Could you check a few things on this model? Use its own coordinates, in mm. A direction names the side the tool comes from. Give positions to 0.01 mm unless a question says otherwise; leave off trailing zeros. Return JSON: item names as keys, results as strings. Group by question number.
```python
from build123d import *

# Parameters (mm, degrees)
SKETCH1_W                    = 106
SKETCH1_H                    = 106
MAINOUTLINE_DEPTH            = 1.6
SKETCH4_W                    = 11.7
SKETCH4_H                    = 11.7
RAILCUTOUTS_DEPTH            = 75.970394157
SKETCH13_W                   = 5.7
SKETCH13_H                   = 1.9
SKETCH13_W_2                 = 1.8
SKETCH13_H_2                 = 3
FILLETCUTOUTS_DEPTH          = 75.970394157
SMOOTHCORNER_DEPTH           = 10
MIRROR2_COPY_1_SKETCH_W      = 11.7
MIRROR2_COPY_1_SKETCH_H      = 11.7
MIRROR2_COPY_1_DEPTH         = 75.970394157
MIRROR2_COPY_2_SKETCH_W      = 5.7
MIRROR2_COPY_2_SKETCH_H      = 1.9
MIRROR2_COPY_2_SKETCH_W_2    = 1.8
MIRROR2_COPY_2_SKETCH_H_2    = 3
MIRROR2_COPY_2_DEPTH         = 75.970394157
MIRROR2_COPY_3_DEPTH         = 10
MIRROR2_COPY_4_SKETCH_W      = 11.7
MIRROR2_COPY_4_SKETCH_H      = 11.7
MIRROR2_COPY_4_DEPTH         = 75.970394157
MIRROR2_COPY_5_SKETCH_W      = 5.7
MIRROR2_COPY_5_SKETCH_H      = 1.9
MIRROR2_COPY_5_SKETCH_W_2    = 1.8
MIRROR2_COPY_5_SKETCH_H_2    = 3
MIRROR2_COPY_5_DEPTH         = 75.970394157
FILLET10_R                   = 0.5
M2_CLEARANCE_HOLE1_D         = 2.1
SKETCH16_W                   = 90
SKETCH16_H                   = 5.2
SKETCH16_W_2                 = 5.2
SKETCH16_H_2                 = 90
CUT_EXTRUDE6_DEPTH           = 0.001
CUT_EXTRUDE8_DEPTH           = 10
SKETCH29_R                   = 0.8
CONNECTOR_LOCATION_DEPTH     = 10
CUT_EXTRUDE_THIN1_DEPTH      = 75.970394157
CUT_EXTRUDE_THIN1_DEPTH_BACK = 75.970394157
SKETCH31_W                   = 125.6
SKETCH31_H                   = 125.6
SKETCH31_W_2                 = 105.6
SKETCH31_H_2                 = 105.6
FILLET12_R                   = 0.5


with BuildPart() as part:
    # Sketch1 → mainOutline (new body)
    with BuildSketch(Plane.XY):
        Rectangle(SKETCH1_W, SKETCH1_H)
    extrude(amount=MAINOUTLINE_DEPTH)

    # Sketch4 → railCutouts (cut, through all)
    with BuildSketch(Plane(origin=(0, 0, 0), x_dir=(-1, 0, 0), z_dir=(0, 0, -1))):
        with Locations((47.15, 47.15)):
            Rectangle(SKETCH4_W, SKETCH4_H)
    railcutouts = extrude(amount=-RAILCUTOUTS_DEPTH, mode=Mode.SUBTRACT)

    # Sketch13 → filletCutouts (cut, symmetric)
    with BuildSketch(Plane(origin=(0, 0, 0), x_dir=(-1, 0, 0), z_dir=(0, 0, -1))):
        with Locations((50.15, 40.35)):
            Rectangle(SKETCH13_W, SKETCH13_H)
        with Locations((40.4, 51.5)):
            Rectangle(SKETCH13_W_2, SKETCH13_H_2)
    filletcutouts = extrude(amount=FILLETCUTOUTS_DEPTH, both=True, mode=Mode.SUBTRACT)

    # Sketch27 → smoothCorner (cut)
    with BuildSketch(Plane.XY.offset(1.6)):
        with BuildLine():
            Line((-40.928025612, 42.198025612), (-40.928025612, 49.628025612))
            Line((-40.928025612, 49.628025612), (-40.398025612, 49.628025612))
            ThreePointArc((-40.398025612, 49.628025612), (-39.5, 50), (-39.128025612, 50.898025612))
            Line((-39.128025612, 50.898025612), (-39.128025612, 53))
            Line((-39.128025612, 53), (-53, 53))
            Line((-53, 53), (-53, 39.028025612))
            Line((-53, 39.028025612), (-48.198025612, 39.028025612))
            ThreePointArc((-48.198025612, 39.028025612), (-47.3, 39.4), (-46.928025612, 40.298025612))
            Line((-46.928025612, 40.298025612), (-46.928025612, 40.928025612))
            Line((-46.928025612, 40.928025612), (-42.198025612, 40.928025612))
            ThreePointArc((-42.198025612, 40.928025612), (-41.3, 41.3), (-40.928025612, 42.198025612))
        make_face()
    smoothcorner = extrude(amount=-SMOOTHCORNER_DEPTH, mode=Mode.SUBTRACT)

    # Mirror1: railCutouts, filletCutouts, smoothCorner across plane
    add(railcutouts.mirror(Plane(origin=(0, 0, 0), x_dir=(0, 0, 1), z_dir=(1, 0, 0))), mode=Mode.SUBTRACT)
    add(filletcutouts.mirror(Plane(origin=(0, 0, 0), x_dir=(0, 0, 1), z_dir=(1, 0, 0))), mode=Mode.SUBTRACT)
    add(smoothcorner.mirror(Plane(origin=(0, 0, 0), x_dir=(0, 0, 1), z_dir=(1, 0, 0))), mode=Mode.SUBTRACT)

    # Mirror2: smoothCorner across plane
    add(smoothcorner.mirror(Plane.ZX), mode=Mode.SUBTRACT)

    # Mirror2 copy 1 sketch → Mirror2 copy 1 (cut, through all)
    with BuildSketch(Plane(origin=(0, 0, 0), x_dir=(1, 0, 0), z_dir=(0, 0, -1))):
        with Locations((47.15, 47.15)):
            Rectangle(MIRROR2_COPY_1_SKETCH_W, MIRROR2_COPY_1_SKETCH_H)
    extrude(amount=-MIRROR2_COPY_1_DEPTH, mode=Mode.SUBTRACT)

    # Mirror2 copy 2 sketch → Mirror2 copy 2 (cut, symmetric)
    with BuildSketch(Plane(origin=(0, 0, 0), x_dir=(1, 0, 0), z_dir=(0, 0, -1))):
        with Locations((50.15, 40.35)):
            Rectangle(MIRROR2_COPY_2_SKETCH_W, MIRROR2_COPY_2_SKETCH_H)
        with Locations((40.4, 51.5)):
            Rectangle(MIRROR2_COPY_2_SKETCH_W_2, MIRROR2_COPY_2_SKETCH_H_2)
    extrude(amount=MIRROR2_COPY_2_DEPTH, both=True, mode=Mode.SUBTRACT)

    # Mirror2 copy 3 sketch → Mirror2 copy 3 (cut)
    with BuildSketch(Plane(origin=(0, 0, 1.6), x_dir=(-1, 0, 0), z_dir=(0, 0, 1))):
        with BuildLine():
            Line((-40.928025612, 42.198025612), (-40.928025612, 49.628025612))
            Line((-40.928025612, 49.628025612), (-40.398025612, 49.628025612))
            ThreePointArc((-40.398025612, 49.628025612), (-39.5, 50), (-39.128025612, 50.898025612))
            Line((-39.128025612, 50.898025612), (-39.128025612, 53))
            Line((-39.128025612, 53), (-53, 53))
            Line((-53, 53), (-53, 39.028025612))
            Line((-53, 39.028025612), (-48.198025612, 39.028025612))
            ThreePointArc((-48.198025612, 39.028025612), (-47.3, 39.4), (-46.928025612, 40.298025612))
            Line((-46.928025612, 40.298025612), (-46.928025612, 40.928025612))
            Line((-46.928025612, 40.928025612), (-42.198025612, 40.928025612))
            ThreePointArc((-42.198025612, 40.928025612), (-41.3, 41.3), (-40.928025612, 42.198025612))
        make_face()
    extrude(amount=-MIRROR2_COPY_3_DEPTH, mode=Mode.SUBTRACT)

    # Mirror2 copy 4 sketch → Mirror2 copy 4 (cut, through all)
    with BuildSketch(Plane(origin=(0, 0, 0), x_dir=(-1, 0, 0), z_dir=(0, 0, -1))):
        with Locations((47.15, -47.15)):
            Rectangle(MIRROR2_COPY_4_SKETCH_W, MIRROR2_COPY_4_SKETCH_H)
    extrude(amount=-MIRROR2_COPY_4_DEPTH, mode=Mode.SUBTRACT)

    # Mirror2 copy 5 sketch → Mirror2 copy 5 (cut, symmetric)
    with BuildSketch(Plane(origin=(0, 0, 0), x_dir=(-1, 0, 0), z_dir=(0, 0, -1))):
        with Locations((50.15, -40.35)):
            Rectangle(MIRROR2_COPY_5_SKETCH_W, MIRROR2_COPY_5_SKETCH_H)
        with Locations((40.4, -51.5)):
            Rectangle(MIRROR2_COPY_5_SKETCH_W_2, MIRROR2_COPY_5_SKETCH_H_2)
    extrude(amount=MIRROR2_COPY_5_DEPTH, both=True, mode=Mode.SUBTRACT)

    # Fillet10
    fillet10_edges = [part.edges().sort_by_distance(p)[0] for p in [
        (40.928025612, 49.628025612, 0.8),
        (46.928025612, 40.928025612, 0.8),
        (46.928025612, -40.928025612, 0.8),
        (40.928025612, -49.628025612, 0.8),
        (-40.928025612, -49.628025612, 0.8),
        (-46.928025612, -40.928025612, 0.8),
        (-46.928025612, 40.928025612, 0.8),
        (-40.928025612, 49.628025612, 0.8),
    ]]
    fillet(fillet10_edges, radius=FILLET10_R)

    # M2 Clearance Hole1 (through all)
    with Locations(Plane(origin=(0, 0, 0), x_dir=(-1, 0, 0), z_dir=(0, 0, -1))):
        with Locations((49.5, -27.5), (27.5, -49.5), (-49.5, -27.5), (-27.5, -49.5), (-27.5, 49.5), (-49.5, 27.5), (27.5, 49.5), (49.5, 27.5)):
            Hole(M2_CLEARANCE_HOLE1_D / 2)

    # Sketch16 → Cut-Extrude6 (cut)
    with BuildSketch(Plane.XY.offset(1.6)):
        with Locations((0, -50.4)):
            Rectangle(SKETCH16_W, SKETCH16_H)
        with Locations((0, 50.4)):
            Rectangle(SKETCH16_W, SKETCH16_H)
        with Locations((-50.4, 0)):
            Rectangle(SKETCH16_W_2, SKETCH16_H_2)
        with Locations((50.4, 0)):
            Rectangle(SKETCH16_W_2, SKETCH16_H_2)
    extrude(amount=-CUT_EXTRUDE6_DEPTH, mode=Mode.SUBTRACT)

    # Sketch30 → Cut-Extrude8 (cut)
    with BuildSketch(Plane(origin=(0, 0, 0), x_dir=(-1, 0, 0), z_dir=(0, 0, -1))):
        with BuildLine():
            Line((-18.930017367, -39.330048004), (-2.75, -23.150030637))
            Line((-2.75, -23.150030637), (2.75, -23.150030637))
            Line((2.75, -23.150030637), (18.930017367, -39.330048004))
            ThreePointArc((18.930017367, -39.330048004), (32.985735805, -32.985735805), (39.330048004, -18.930017367))
            Line((39.330048004, -18.930017367), (23.150030637, -2.75))
            Line((23.150030637, -2.75), (23.150030637, 2.75))
            Line((23.150030637, 2.75), (39.330048004, 18.930017367))
            ThreePointArc((39.330048004, 18.930017367), (32.985735805, 32.985735805), (18.930017367, 39.330048004))
            Line((18.930017367, 39.330048004), (2.75, 23.150030637))
            Line((2.75, 23.150030637), (-2.75, 23.150030637))
            Line((-2.75, 23.150030637), (-18.930017367, 39.330048004))
            ThreePointArc((-18.930017367, 39.330048004), (-32.985735805, 32.985735805), (-39.330048004, 18.930017367))
            Line((-39.330048004, 18.930017367), (-23.150030637, 2.75))
            Line((-23.150030637, 2.75), (-23.150030637, -2.75))
            Line((-23.150030637, -2.75), (-39.330048004, -18.930017367))
            ThreePointArc((-39.330048004, -18.930017367), (-32.985735805, -32.985735805), (-18.930017367, -39.330048004))
        make_face()
    extrude(amount=-CUT_EXTRUDE8_DEPTH, mode=Mode.SUBTRACT)

    # Sketch29 → Connector Location (cut)
    with BuildSketch(Plane(origin=(0, 0, 0), x_dir=(-1, 0, 0), z_dir=(0, 0, -1))):
        with Locations((34.285, -42.5)):
            Circle(SKETCH29_R)
        with Locations((23.515, -42.5)):
            Circle(SKETCH29_R)
    extrude(amount=-CONNECTOR_LOCATION_DEPTH, mode=Mode.SUBTRACT)

    # Sketch31 → Cut-Extrude-Thin1 (cut, two sides: drawn at the far end of the back side and taken through both)
    with BuildSketch(Plane(origin=(0, 0, 0), x_dir=(-1, 0, 0), z_dir=(0, 0, -1)).offset(-CUT_EXTRUDE_THIN1_DEPTH_BACK)):
        Rectangle(SKETCH31_W, SKETCH31_H)
        Rectangle(SKETCH31_W_2, SKETCH31_H_2, mode=Mode.SUBTRACT)
    extrude(amount=CUT_EXTRUDE_THIN1_DEPTH + CUT_EXTRUDE_THIN1_DEPTH_BACK, mode=Mode.SUBTRACT)

    # Fillet12
    fillet12_edges = [part.edges().sort_by_distance(p)[0] for p in [
        (-52.8, 39.028025612, 0.7995),
        (39.128025612, -52.8, 0.7995),
        (52.8, -39.028025612, 0.7995),
        (-39.128025612, 52.8, 0.7995),
        (-52.8, -39.028025612, 0.7995),
        (-39.128025612, -52.8, 0.7995),
        (52.8, 39.028025612, 0.7995),
        (39.128025612, 52.8, 0.7995),
    ]]
    fillet(fillet12_edges, radius=FILLET12_R)


solid = part.part
```
1. I need wall thicknesses on L1, parallel to Y at x = 49.5, z = 1.05; L2, parallel to Y at x = 1, z = 0.15; L3, parallel to Y at x = 27.5, z = 1.25. Which ranges of each line are inside material? Lowest first, please. Write a range as from..to.
2. If we mould it in two halves opening along X, with no side actions, what happens to faces 3 (the flat face through (11, -31.4, 0.8)), 4 (the flat face through (-1, 50, 1.599))? For each: pulls with the +X half, pulls with the -X half, needs draft (parallel to the pull), parting line crosses it, or undercut.
3. Imagine slicing it at C-C, the plane x = 35. Count the separate pieces of the cut face and the enclosed holes in it, plus the area to 3 significant figures.
4. For pin 1 (0.5 mm diameter, centred on x = -49.5, z = 0.5, fed in from -Y); pin 2 (1.9 mm diameter, centred on x = 27.5, y = -49.5, fed in from +Z), each with a flat end and sliding along its axis, tell me the tip position at first contact or that it passes through.
5. Which directions (+Z, -Z, +X, -X, +Y, -Y) give clear straight access to the entire face, cutting with the end or side of a thin tool? Please do faces 1 (the cylindrical face through (33.14, -32.83, 0.79)), 2 (the flat face through (-50, 1, 1.599)).
Values:
{
 "1": {"L1": "y = -39.03..-28.55, -26.45..26.45, 28.55..39.03", "L2": "y = -52.8..-23.15, 23.15..52.8", "L3": "y = -52.8..-50.55, -48.45..-36.98, -7.1..7.1, 36.98..48.45, 50.55..52.8"},
 "2": {"face 3": "undercut", "face 4": "needs draft"},
 "3": {"separate pieces": "3", "enclosed holes": "0", "area": "118 mm²"},
 "4": {"pin 1": "stops at y = -39.03", "pin 2": "passes through"},
 "5": {"face 1": "+Z, -Z", "face 2": "+Z, +X, -X, +Y, -Y"}
}
